```python
from build123d import *

# Parameters (mm, degrees)
SKETCH1_R           = 10.16
SKETCH1_R_2         = 6.35
BOSS_EXTRUDE2_DEPTH = 20.828
BOSS_EXTRUDE3_START = 12.7
SKETCH2_R           = 10.16
SKETCH2_R_2         = 8.001
BOSS_EXTRUDE3_DEPTH = 12.7
SKETCH3_R           = 10.16
SKETCH3_R_2         = 8.001
BOSS_EXTRUDE4_DEPTH = 12.7


with BuildPart() as part:
    # Sketch1 → Boss-Extrude2 (new body)
    with BuildSketch(Plane(origin=(0, 0, 0), x_dir=(0, 0, -1), z_dir=(1, 0, 0))):
        Circle(SKETCH1_R)
        Circle(SKETCH1_R_2, mode=Mode.SUBTRACT)
    extrude(amount=BOSS_EXTRUDE2_DEPTH)

    # Sketch2 → Boss-Extrude3 (add)
    with BuildSketch(Plane.ZY.offset(BOSS_EXTRUDE3_START)):
        Circle(SKETCH2_R)
        Circle(SKETCH2_R_2, mode=Mode.SUBTRACT)
    extrude(amount=-BOSS_EXTRUDE3_DEPTH)

    # Sketch3 → Boss-Extrude4 (add)
    with BuildSketch(Plane(origin=(20.828, 0, 0), x_dir=(0, 0, -1), z_dir=(1, 0, 0))):
        with Locations(Location((0, 0, 0), (0, 0, 180))):
            Circle(SKETCH3_R)
        with Locations(Location((0, 0, 0), (0, 0, 180))):
            Circle(SKETCH3_R_2, mode=Mode.SUBTRACT)
    extrude(amount=BOSS_EXTRUDE4_DEPTH)


solid = part.part
```
Design review of the part built by this model. Coordinates are the model's own, in mm. Coordinates: 2 decimals unless noted, no trailing zeros. Loops run counter-clockwise (first coordinate to the right, second up) from the corner with the lowest first, then second, coordinate; pieces in that order, holes last. Notation, with made-up numbers: M 48,29 L 52,29 A22 ccw 52,35 Z; hole C -17.75,69.5 d1. An arc over 180 degrees is marked long. One line per question, with ' | ' between items.
(1) We need section D-D (y = -7.25). Give the boundary of the cut face in (x, z), and give its area (3 significant figures).
Filled in:
outline: M -12.7,-7.12 L 33.53,-7.12 L 33.53,-3.38 L 20.83,-3.38 L 20.83,3.38 L 33.53,3.38 L 33.53,7.12 L -12.7,7.12 L -12.7,3.38 L 0,3.38 L 0,-3.38 L -12.7,-3.38 Z | area: 486 mm^2
(2) We need section C-C (x = 29). Give the boundary of the cut face in (y, z).
Filled in:
outline: C 0,0 d20.32; hole C 0,0 d16
(3) Wall thickness on probe 1 along Y at (x, z) = (30, 0); probe 2 along Y at (x, z) = (9, 0): over which ranges is each line inside the solid? List them lowest first.
Filled in:
probe 1: y = -10.16 to -8, 8 to 10.16 | probe 2: y = -10.16 to -6.35, 6.35 to 10.16
(4) We need section A-A (y = 0). Give the boundary of the cut face in (x, z).
Filled in:
outline: M -12.7,-10.16 L 33.53,-10.16 L 33.53,-8 L 20.83,-8 L 20.83,-6.35 L 0,-6.35 L 0,-8 L -12.7,-8 Z; M -12.7,8 L 0,8 L 0,6.35 L 20.83,6.35 L 20.83,8 L 33.53,8 L 33.53,10.16 L -12.7,10.16 Z
(5) Draft analysis for pull direction Y (two halves, no side actions). For faces 1 (the face through (-6.44, -7.81, -1.73)), 2 (the face through (27.09, 7.81, -1.73)), 3 (the face through (-12.7, -8.2, 0)), state which applies: released by +Y, released by -Y, zero draft, split by the parting line, or undercut.
Filled in:
face 1: undercut | face 2: undercut | face 3: zero draft
(6) For pin 1 Ø12 at (x, y) = (10, -6.5) entering from -Z; pin 2 Ø3 at (x, y) = (18.5, -7.5) entering from -Z; pin 3 Ø1 at (y, z) = (-2, -7) entering from +X; pin 4 Ø10 at (x, z) = (20, -4) entering from -Y, all flat-tipped, find the tip position at first contact; note any pin that passes through.
Filled in:
pin 1: stops at z = -10.15 | pin 2: stops at z = -8.2 | pin 3: stops at x = 20.83 | pin 4: stops at y = -10.16
